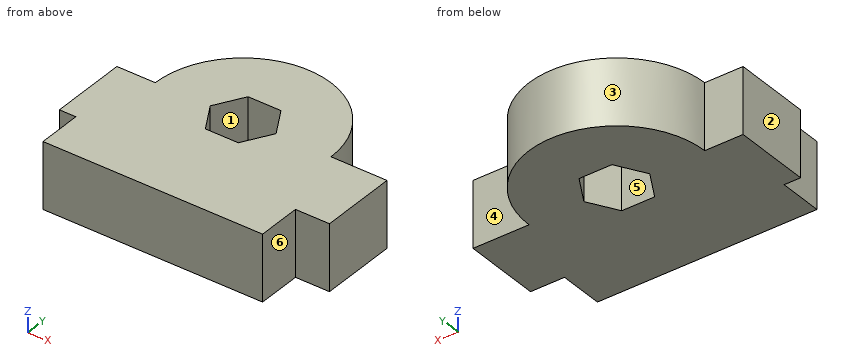
from build123d import *

# Parameters (mm, degrees)
BOSS_EXTRUDE1_DEPTH = 6


with BuildPart() as part:
    # Sketch1 → Boss-Extrude1 (new body)
    with BuildSketch(Plane.XY):
        with BuildLine():
            Line((0, 0), (20, 0))
            Line((20, 0), (20, 4))
            Line((20, 4), (23.1, 4))
            Line((23.1, 4), (23.1, 11))
            Line((23.1, 11), (18, 11))
            ThreePointArc((18, 11), (10, 19), (2, 11))
            Line((2, 11), (-1.5, 11))
            Line((-1.5, 11), (-1.5, 4))
            Line((-1.5, 4), (0, 4))
            Line((0, 4), (0, 0))
        make_face()
        Polygon((13, 11), (11.5, 13.598076211), (8.5, 13.598076211), (7, 11), (8.5, 8.401923789), (11.5, 8.401923789), align=None, mode=Mode.SUBTRACT)
    extrude(amount=BOSS_EXTRUDE1_DEPTH)


solid = part.part
Build history of the part. All positions in model axes, mm. Face numbers are marked on the shaded views. A direction names the side the tool comes from. Give positions to 0.01 mm unless a question says otherwise; leave off trailing zeros. Order: outer loops, then holes, each group sorted by start corner. A loop starts at its lowest first (then second) coordinate and runs counter-clockwise, first axis right, second up. Notation, with made-up numbers: M 37,62 L 80,62 A27 ccw 80,79 Z; hole C 4.25,24.25 d1. An arc over 180 degrees is marked long. Use one line per item in the form item = value.
1) Saw through at C-C (z = 5.25). Give the cut face in (x, y), plus the area to 3 significant figures.
Calculated:
outline = M -1.5,4 L 0,4 L 0,0 L 20,0 L 20,4 L 23.1,4 L 23.1,11 L 18,11 A8 ccw 2,11 L -1.5,11 Z; hole M 7,11 L 8.5,8.4 L 11.5,8.4 L 13,11 L 11.5,13.6 L 8.5,13.6 Z
area = 329 mm2
2) Probe probe 1 along X at (y, z) = (9.75, 0.8); probe 2 along Y at (x, z) = (19.5, 1.9); probe 3 along X at (y, z) = (12.5, 5.7). List the from-to ranges inside material, lowest first.
Calculated:
probe_1 = -1.5 to 7.72, 12.28 to 23.1
probe_2 = 0 to 11
probe_3 = 2.14 to 7.87, 12.13 to 17.86
3) Saw through at D-D (x = 21.25). Give the cut face in (y, z), plus the area to 3 significant figures.
Calculated:
outline = M 4,0 L 11,0 L 11,6 L 4,6 Z
area = 42.0 mm2
4) Drop flat-ended pins along their axis: pin 1 (6 mm diameter, centred on x = 8.5, y = 5, fed in from -Z); pin 2 (0.9 mm diameter, centred on x = 22, z = 4, fed in from -Y); pin 3 (1.5 mm diameter, centred on x = 9, z = 2, fed in from +Y). Give the stop position or say it passes through.
Calculated:
pin_1 = 0
pin_2 = 4
pin_3 = 19
5) Saw through at B-B (y = 11.75). Give the cut face in (x, z), plus the area to 3 significant figures.
Calculated:
outline = M 2.04,0 L 7.43,0 L 7.43,6 L 2.04,6 Z; M 12.57,0 L 17.96,0 L 17.96,6 L 12.57,6 Z
area = 64.8 mm2
6) Two-plate mould, pull along X, no slides. Class the marked faces 1, 2 and 3: released by +X, released by -X, zero draft, split by the parting line, or undercut.
Calculated:
face_1 = undercut
face_2 = released by -X
face_3 = split by the parting line
7) Saw through at A-A (x = 10). Give the cut face in (y, z), plus the area to 3 significant figures.
Calculated:
outline = M 0,0 L 8.4,0 L 8.4,6 L 0,6 Z; M 13.6,0 L 19,0 L 19,6 L 13.6,6 Z
area = 82.8 mm2
8) Tool access for the marked faces 4, 5 and 6: list every direction of +Z, -Z, +X, -X, +Y, -Y with a clear straight run to the whole face (end or side of a thin tool).
Calculated:
face_4 = +Z, -Z, +X, +Y
face_5 = +Z, -Z
face_6 = +Z, -Z, +X, -Y
